Read the model definition and answer for the solid it produces. Units are mm, in the model's axes. Give positions to 0.01 mm unless a question says otherwise; leave off trailing zeros. Loops run counter-clockwise (first coordinate to the right, second up) from the corner with the lowest first, then second, coordinate; pieces in that order, holes last. Notation, with made-up numbers: (75, 72.25) - (102, 72.25) arc R10 cw to (102, 87.25) - close; hole circle Ø11 at (-17, -12). An arc over 180 degrees is marked (long way). Use a Markdown table: item, result. Add a question column.
Item 1: A cutting plane is placed at A-A (y = 2.75). Determine the outline of the cut face in (x, z).
Item 2: A cutting plane is placed at B-B (z = 195.5). Determine the outline of the cut face in (x, y), plus the area to 3 significant figures.
Item 3: Consider probe 1 along Y at (x, z) = (-2, 34.5); probe 2 along X at (y, z) = (6.2, 295); probe 3 along X at (y, z) = (-17.25, 147.5). Determine where each line is inside the solid, lowest interval first. Write a range as [from, to].
Autodesk Inventor part; units mm, degrees
ref_plane "YZ Plane" through (0, 0, 0) normal (1, 0, 0) x (0, 1, 0)
ref_plane "XZ Plane" through (0, 0, 0) normal (0, 1, 0) x (-1, 0, 0)
ref_plane "XY Plane" through (0, 0, 0) normal (0, 0, 1) x (1, 0, 0)
sketch "スケッチ1" plane through (0, 0, 0) normal (0, 0, 1) x (1, 0, 0)
  line L0 (-11.3154, 7.0975) -> (3.6846, 7.0975)
  line L1 (3.6846, 7.0975) -> (3.6846, -22.9025)
  line L2 (3.6846, -22.9025) -> (-11.3154, -22.9025)
  line L3 (-11.3154, -22.9025) -> (-11.3154, 7.0975)
  point P0 (0, 0)
  dimension "d0" = 15
  dimension "d1" = 30
extrude "押し出し1" add sketch "スケッチ1" along normal blind 330
sketch "スケッチ2" plane through (3.6846, -22.9025, 0) normal (1, 0, 0) x (0, 0, -1)
  circle A0 centre (-320, 15) radius 1.5
  line L0 (0, 30) -> (-330, 30)
  line L1 (-330, 0) -> (-330, 30)
  circle A1 centre (-310, 15) radius 1.5
  circle A2 centre (-300, 15) radius 1.5
  circle A3 centre (-30, 15) radius 1.5
  circle A4 centre (-20, 15) radius 1.5
  circle A5 centre (-10, 15) radius 1.5
  line L2 (0, 30) -> (0, 0)
  point P0 (0, 22.9025)
  dimension "d4" = 3
  dimension "d5" = 15
  dimension "d6" = 10
  dimension "d7" = 3
  dimension "d8" = 3
  dimension "d9" = 3
  dimension "d10" = 3
  dimension "d11" = 3
  dimension "d12" = 10
  dimension "d13" = 10
  dimension "d14" = 10
  dimension "d15" = 10
  dimension "d16" = 10
hole "穴1" at (3.6846, -7.9025, 320) at (3.6846, -7.9025, 310) at (3.6846, -7.9025, 300) at (3.6846, -7.9025, 10) at (3.6846, -7.9025, 20) at (3.6846, -7.9025, 30) direction (-1, 0, 0) diameter 3 depth 15
sketch "スケッチ3" plane through (-11.3154, 7.0975, 0) normal (0, 1, 0) x (1, 0, 0)
  circle A0 centre (7.5, -15) radius 1.5
  line L0 (0, 0) -> (15, 0)
  circle A1 centre (7.5, -25) radius 1.5
  circle A2 centre (7.5, -35) radius 1.5
  circle A3 centre (7.5, -315) radius 1.5
  line L1 (15, -330) -> (0, -330)
  circle A4 centre (7.5, -305) radius 1.5
  circle A5 centre (7.5, -295) radius 1.5
  point P0 (11.3154, 0)
  dimension "d24" = 3
  dimension "d25" = 15
  dimension "d26" = 3
  dimension "d27" = 3
  dimension "d28" = 3
  dimension "d29" = 15
  dimension "d30" = 3
  dimension "d31" = 3
  dimension "d32" = 10
  dimension "d33" = 10
  dimension "d34" = 10
  dimension "d35" = 10
hole "穴2" at (-3.8154, 7.0975, 295) at (-3.8154, 7.0975, 305) at (-3.8154, 7.0975, 315) at (-3.8154, 7.0975, 15) at (-3.8154, 7.0975, 25) at (-3.8154, 7.0975, 35) direction (0, -1, 0) diameter 3 depth 30
sketch "スケッチ4" plane through (0, 0, 330) normal (0, 0, 1) x (1, 0, 0)
  line L0 (-9.8154, 5.5975) -> (2.1846, 5.5975)
  line L1 (2.1846, 5.5975) -> (2.1846, -21.4025)
  line L2 (2.1846, -21.4025) -> (-9.8154, -21.4025)
  line L3 (-9.8154, -21.4025) -> (-9.8154, 5.5975)
  line L4 (3.6846, 7.0975) -> (-11.3154, 7.0975)
  line L5 (-11.3154, 7.0975) -> (-11.3154, -22.9025)
  point P0 (0, 0)
  dimension "d43" = 12
  dimension "d44" = 27
  dimension "d45" = 1.5
  dimension "d46" = 1.5
extrude "押し出し2" cut sketch "スケッチ4" against normal blind 330
equation "\"BendRadius\" = Thickness"
equation "\"BendReliefWidth\" = Thickness"
equation "\"BendReliefDepth\" = 0.5 * Thickness"
equation "\"CornerReliefSize\" = 4 * Thickness"
equation "\"MinimumRemnant\" = 2 * Thickness"
equation "\"TransitionRadius\" = BendRadius"
equation "\"JacobiRadiusSize\" = BendRadius"
equation "\"GapSize\" = Thickness"
properties part number "nhk15" material "アルミニウム 6061"
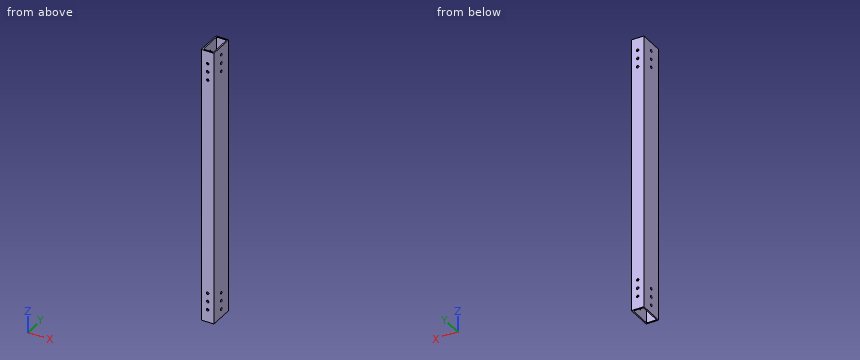
Geometry says:
| question | item | result |
|---|---|---|
| 1 | outline | (-11.32, 0) - (-9.82, 0) - (-9.82, 330) - (-11.32, 330) - close; (2.18, 0) - (3.68, 0) - (3.68, 330) - (2.18, 330) - close |
| 2 | outline | (-11.32, -22.9) - (3.68, -22.9) - (3.68, 7.1) - (-11.32, 7.1) - close; hole (-9.82, -21.4) - (2.18, -21.4) - (2.18, 5.6) - (-9.82, 5.6) - close |
| 2 | area | 126 mm² |
| 3 | probe 1 | [-22.9, -21.4], [5.6, 7.1] |
| 3 | probe 2 | [-11.32, -5.32], [-2.32, 3.68] |
| 3 | probe 3 | [-11.32, -9.82], [2.18, 3.68] |
